Geometry check sheet. Reference: the model listing, model coordinates, mm. A direction names the side the tool comes from. Coordinates: 2 decimals unless noted, no trailing zeros. Loops run counter-clockwise (first coordinate to the right, second up) from the corner with the lowest first, then second, coordinate; pieces in that order, holes last. Notation, with made-up numbers: M -40,89.25 L -28,89.25 A32 cw -28,126.25 Z; hole C 31.5,-25 d2. An arc over 180 degrees is marked long. One line per question, with ' | ' between items. Start each with the question number.
Autodesk Inventor part; units mm, degrees
ref_plane "YZ Plane" through (0, 0, 0) normal (1, 0, 0) x (0, 1, 0)
ref_plane "XZ Plane" through (0, 0, 0) normal (0, 1, 0) x (-1, 0, 0)
ref_plane "XY Plane" through (0, 0, 0) normal (0, 0, 1) x (1, 0, 0)
sketch "Sketch1" plane through (0, 0, 0) normal (0, 1, 0) x (-1, 0, 0)
  line L0 (56, 0) -> (-56, 0)
  line L1 (0, -35) -> (0, 35)
  line L2 (40, 25) -> (-40, 25)
  line L3 (-40, 25) -> (-40, -25)
  line L4 (-40, -25) -> (40, -25)
  line L5 (40, -25) -> (40, 25)
  point P0 (0, 0)
  point P1 (40, 0)
  point P2 (0, -25)
  dimension "d0" = 50
  dimension "d1" = 80
extrude "Extrusion1" add sketch "Sketch1" along normal blind 15
sketch "Sketch2" plane through (40, 0, 25) normal (1, 0, 0) x (0, 0, -1)
  line L0 (0, 0) -> (50, 0)
  line L1 (50, 0) -> (50, 15)
  line L2 (0, 15) -> (50, 15)
  line L3 (0, 0) -> (0, 15)
  line L4 (0, 0) -> (50, 0)
  line L5 (50, 0) -> (50, 80)
  line L6 (0, 80) -> (0, 0)
  arc A0 (50, 80) -> (0, 80) centre (25, 80) ccw
  line L7 (0, 0) -> (50, 0)
  circle A1 centre (25, 80) radius 10
  line L8 (25, -19) -> (25, 114)
  point P0 (25, 0)
  dimension "d5" = 50
  dimension "d6" = 20
  dimension "d7" = 80
  dimension "d8" = 50
extrude "Extrusion2" add sketch "Sketch2" against normal blind 15 contours L3 L2 L8 L0 | L8 L2 L1 L0 | L6 A0 L8 A1 L2 | L8 A1 A0 L5 L2
mirror "Mirror1" about plane through (0, 0, 0) normal (1, 0, 0) of "Extrusion2"
properties part number "Base_Block" material "Steel, Carbon"
1. Sectioned sample at B-B (z = 0). Record the cut outline in (x, y).
2. Sectioned sample at C-C (x = -34.5). Record the cut outline in (y, z).
3. Draft check along Y on faces 1 (the cylindrical face through (-32.61, 71.57, -5.38)), 2 (the flat face through (-40, 52, 0)), 3 (the cylindrical face through (-32.605, 104.994, 0.55)). Enter one of: +Y half, -Y half, draft (parallel to the pull), parting line (faces both ways), or undercut.
4. Sectioned sample at A-A (y = 67). Record the cut outline in (x, z).
5. Thickness scan on line 1 (Z direction, x = 28.75, y = 80); line 2 (X direction, y = 49, z = -2); line 3 (Y direction, x = -29.5, z = 0). Record the ranges inside material, lowest first.
6. Tool access check on faces 4 (the flat face through (-25, 61, 0)), 5 (the flat face through (1, 13, -25)). Record the directions out of +Z, -Z, +X, -X, +Y, -Y that give a thin tool (end or side, any length) a straight path to the whole face; none if there is none.
7. Sectioned sample at D-D (z = -16). Record the cut outline in (x, y), and give its area (3 significant figures).
8. Depth check by flat-ended pin: pin 1 Ø10 at (x, y) = (21, 46) entering from -Z; pin 2 Ø15 at (x, z) = (7.5, -11.5) entering from +Y. Enter the tip coordinate at first touch or a pass-through.
Result:
1) outline: M -40,0 L 40,0 L 40,70 L 25,70 L 25,15 L -25,15 L -25,70 L -40,70 Z; M -40,90 L -25,90 L -25,105 L -40,105 Z; M 25,90 L 40,90 L 40,105 L 25,105 Z
2) outline: M 0,-25 L 80,-25 A25 ccw 80,25 L 0,25 Z; hole C 80,0 d20
3) face 1: undercut | face 2: draft | face 3: +Y half
4) outline: M -40,-25 L -25,-25 L -25,25 L -40,25 Z; M 25,-25 L 40,-25 L 40,25 L 25,25 Z
5) line 1: z = -25 to -10, 10 to 25 | line 2: x = -40 to -25, 25 to 40 | line 3: y = 0 to 70, 90 to 105
6) face 4: +Z, -Z, +Y | face 5: -Z, +X, -X, +Y, -Y
7) outline: M -40,0 L 40,0 L 40,99.21 L 25,99.21 L 25,15 L -25,15 L -25,99.21 L -40,99.21 Z | area: 3,730 mm2
8) pin 1: stops at z = -25 | pin 2: stops at y = 15
